Source: CAD feature listing. Evaluate the final solid. Frame: model axes, mm. A direction names the side the tool comes from. Give positions to 0.01 mm unless a question says otherwise; leave off trailing zeros. Loops run counter-clockwise (first coordinate to the right, second up) from the corner with the lowest first, then second, coordinate; pieces in that order, holes last. Notation, with made-up numbers: (78.25, -5) -> (115.25, -5) arc R18 ccw to (115.25, 1) -> close; hole circle Ø10 at (-11.75, 20.5). An arc over 180 degrees is marked (long way). Put each result on its own line as item: value.
Autodesk Inventor part; units mm, degrees
ref_plane "YZ Plane" through (0, 0, 0) normal (1, 0, 0) x (0, 1, 0)
ref_plane "XZ Plane" through (0, 0, 0) normal (0, 1, 0) x (-1, 0, 0)
ref_plane "XY Plane" through (0, 0, 0) normal (0, 0, 1) x (1, 0, 0)
sketch "Sketch1" plane through (0, 0, 0) normal (0, 0, 1) x (1, 0, 0)
  circle A0 centre (0, 0) radius 76.2
  dimension "d0" = 152.4
extrude "Extrusion1" add sketch "Sketch1" along normal blind 25.4
sketch "Sketch2" plane through (0, 0, 25.4) normal (0, 0, 1) x (1, 0, 0)
  circle A0 centre (0, 0) radius 76.2
  circle A1 centre (0, 0) radius 38.1
  dimension "d3" = 76.2
extrude "Extrusion2" cut sketch "Sketch2" against normal blind 2.54 contours A1
sketch "Sketch3" plane through (0, 0, 0) normal (0, 0, -1) x (-1, 0, 0)
  circle A0 centre (0, 0) radius 76.2
  circle A1 centre (0, 0) radius 38.1
  dimension "d6" = 76.2
extrude "Extrusion3" cut sketch "Sketch3" against normal blind 2.54 contours A1
fillet "Fillet1" radius 12.7 2 edges at (-76.2, 0, 25.4) (-76.2, 0, 0)
sketch "Sketch4" plane through (0, 0, 22.86) normal (0, 0, 1) x (1, 0, 0)
  circle A0 centre (0, 0) radius 38.1
  circle A1 centre (0, 0) radius 6.35
  dimension "d10" = 12.7
extrude "Extrusion4" add sketch "Sketch4" along normal blind 6.35 contours A1
sketch "Sketch5" plane through (0, 0, 2.54) normal (0, 0, -1) x (-1, 0, 0)
  circle A0 centre (0, 0) radius 38.1
  circle A1 centre (0, 0) radius 6.35
  dimension "d13" = 12.7
extrude "Extrusion5" add sketch "Sketch5" along normal blind 6.35 contours A1
properties part number "wheel"
(1) Draft query along Y for faces 4 (the flat face through (0, 0, -3.81)), 5 (the cylindrical face through (-1.38, 6.2, 25.99)). Return one class per face: released by +Y, released by -Y, zero draft, split by the parting line, or undercut.
Calculated:
face 4: zero draft
face 5: undercut
(2) Line query: probe 1 along Z at (x, y) = (-46.5, 31); probe 2 along Y at (x, z) = (-22, 23); probe 3 along Z at (x, y) = (26, -19). Output: solid intervals per line, ascending. Write a range as from..to.
Calculated:
probe 1: z = 0..25.4
probe 2: y = -67.43..-31.11, 31.11..67.43
probe 3: z = 2.54..22.86
(3) Section C-C on z = 18. Return loops of the section in (x, y).
Calculated:
outline: circle Ø150.08 at (0, 0)
(4) Reachability of faces 1 (the flat face through (0, 0, 29.21)), 2 (the cylindrical face through (1.38, 6.2, -0.59)), 3 (the cylindrical face through (-30.235, -23.183, 24.148)) from +Z, -Z, +X, -X, +Y, -Y: full face, straight path, thin tool, end or side. Return the list, or none.
Calculated:
face 1: +Z, +X, -X, +Y, -Y
face 2: -Z
face 3: +Z
(5) First-contact query: P1, Ø10, axis at x = -15.5, y = -47.5, coming from the -Z side; P2, Ø5, axis at x = 45, y = -55, coming from the -Z side; P3, Ø10, axis at x = 25, z = 9.5, coming from the +Y side; P4, Ø23, axis at x = 10, y = 13.5, coming from the -Z side. Flat tips, straight axial feed; report the tip coordinate or a pass-through.
Calculated:
P1: stops at z = 0
P2: stops at z = 1.05
P3: stops at y = 73.36
P4: stops at z = -3.81
